Verification items for the finished model (mm, model axes). Face numbers are marked on the shaded views. A direction names the side the tool comes from. Coordinates: 2 decimals unless noted, no trailing zeros. Write each loop counter-clockwise with the first axis right and the second up, starting at its lowest first coordinate (ties: lowest second). Pieces come first, ordered by that corner, then holes. Notation, with made-up numbers: (88, 68.25) -> (103, 68.25) arc R21 ccw to (103, 79.25) -> close; hole circle Ø3 at (-37.75, -25.75). An arc over 180 degrees is marked (long way). Use a Markdown table: item, result. Add a question column.
from build123d import *

# Parameters (mm, degrees)
CYLINDER007_R     = 13.9827
CYLINDER007_DEPTH = 64.36
CYLINDER006_R     = 13.9827
CYLINDER006_DEPTH = 31.877


with BuildPart() as cylinder007:
    # Cylinder007 → Cylinder007 (new body)
    with BuildSketch(Plane.XZ.offset(-32.1818)):
        Circle(CYLINDER007_R)
    extrude(amount=CYLINDER007_DEPTH)


with BuildPart() as t:
    # Cylinder006 → Cylinder006 (new body)
    with BuildSketch(Plane.XY):
        Circle(CYLINDER006_R)
    extrude(amount=CYLINDER006_DEPTH)

    # Fusion002: union Cylinder007
    add(cylinder007.part)


solid = t.part
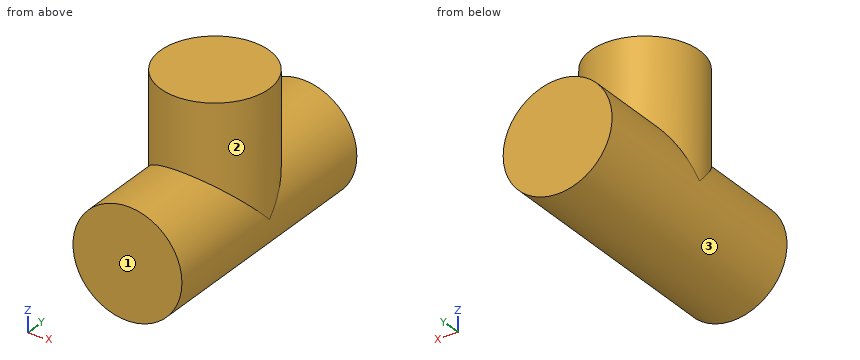
1) Cross-section at A-A on x = 0. Record the boundary of the cut face in (y, z).
2) Cross-section at D-D on y = 0. Record the boundary of the cut face in (x, z).
3) Thickness scan on L1, parallel to Z at x = 0, y = 20; L2, parallel to X at y = 12, z = 14.5; L3, parallel to Y at x = 9.5, z = 24. Record the ranges inside material, lowest first.
4) Gauge pin test, flat ends, axial feed: pin 1 (5 mm diameter, centred on x = 4.5, y = -21.5, fed in from +Z); pin 2 (2 mm diameter, centred on x = 8.5, y = 18.5, fed in from +Z); pin 3 (12 mm diameter, centred on x = -4, z = 21, fed in from -Y). Record the tip position at first contact, or that the pin passes through.
5) Cross-section at C-C on y = 24.5. Record the boundary of the cut face in (x, z), then the cut area to 3 significant figures.
6) Cross-section at B-B on z = 12. Record the boundary of the cut face in (x, y), then the cut area to 3 significant figures.
7) Set-up check for the marked faces 1, 2 and 3: record each of +Z, -Z, +X, -X, +Y, -Y from which the full face is reachable in a straight line by a thin tool's end or side.
Returned:
| question | item | result |
|---|---|---|
| 1 | outline | (-32.18, -13.98) -> (32.18, -13.98) -> (32.18, 13.98) -> (13.98, 13.98) -> (13.98, 31.88) -> (-13.98, 31.88) -> (-13.98, 13.98) -> (-32.18, 13.98) -> close |
| 2 | outline | (-13.98, 0) arc R13.98 ccw to (13.98, 0) -> (13.98, 31.88) -> (-13.98, 31.88) -> close |
| 3 | L1 | z = -13.98 to 13.98 |
| 3 | L2 | x = -7.18 to 7.18 |
| 3 | L3 | y = -10.26 to 10.26 |
| 4 | pin 1 | stops at z = 13.84 |
| 4 | pin 2 | stops at z = 11.8 |
| 4 | pin 3 | stops at y = -13.98 |
| 5 | outline | circle Ø27.97 at (0, 0) |
| 5 | area | 614 mm² |
| 6 | outline | (-7.18, -32.18) -> (7.18, -32.18) -> (7.18, -12) arc R13.98 ccw to (7.18, 12) -> (7.18, 32.18) -> (-7.18, 32.18) -> (-7.18, 12) arc R13.98 ccw to (-7.18, -12) -> close |
| 6 | area | 1,160 mm² |
| 7 | face 1 | +Z, -Z, +X, -X, -Y |
| 7 | face 2 | +Z |
| 7 | face 3 | none |
